Could you check a few things on this drawing? It's one solid part, dimensions in mm from its lowest x, y, z. A direction names the side the tool comes from. Give positions to 0.01 mm unless a question says otherwise; leave off trailing zeros. Loops run counter-clockwise (first coordinate to the right, second up) from the corner with the lowest first, then second, coordinate; pieces in that order, holes last. Notation, with made-up numbers: (-35, 15.25) -> (20, 15.25) arc R15 ccw to (20, 32.25) -> close; hole circle Ø4 at (15.5, 60). An arc over 180 degrees is marked (long way). Use CSV: the item, a comma, the result in double quotes.
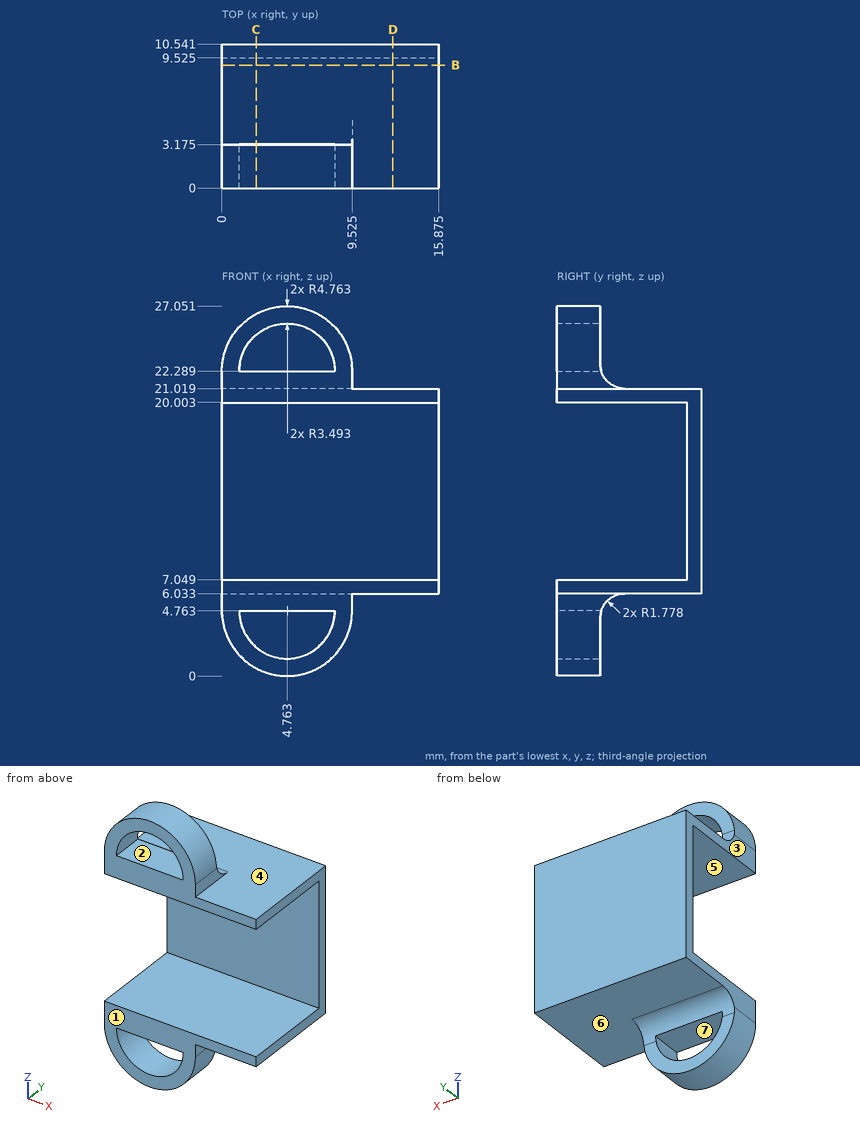
(1) If we section it at B-B, the plane y = 9: Write out the boundary of the cut face in (x, z) (1 decimal).
Answer sheet:
outline,"(0, 6) -> (15.9, 6) -> (15.9, 7) -> (0, 7) -> close; (0, 20) -> (15.9, 20) -> (15.9, 21) -> (0, 21) -> close"
(2) We'd pull the mould along X, two halves only. Please class the marked faces 1, 2 and 3: released by +X, released by -X, zero draft, split by the parting line, or undercut.
Answer sheet:
face 1,"zero draft"
face 2,"undercut"
face 3,"released by -X"
(3) If I drill on L1, parallel to Z at x = 2.25, y = 8; L2, parallel to Y at x = 9.25, z = 13.5 (1 decimal); L3, parallel to Y at x = 8, z = 24.25 (1 decimal), over which ranges is the centre line in solid material (lowest first)? Write a range as from..to.
Answer sheet:
L1,"z = 6.03..7.05, 20..21.02"
L2,"y = 9.5..10.5"
L3,"y = 0..3.2"
(4) Will these pins go through, and if not, where does the flat tip stop? pin 1 Ø5 at (x, y) = (11.5, 6.5) entering from -Z; pin 2 Ø1.5 at (x, z) = (11, 18.5) entering from -Y (1 decimal); pin 3 Ø2 at (x, y) = (6.5, 5) entering from +Z (1 decimal).
Answer sheet:
pin 1,"stops at z = 6.03"
pin 2,"stops at y = 9.5"
pin 3,"stops at z = 21.3"
(5) Which directions (+Z, -Z, +X, -X, +Y, -Y) give clear straight access to the entire face, cutting with the end or side of a thin tool? Please do the marked faces 4, 5, 6 and 7.
Answer sheet:
face 4,"+Z, +X, +Y"
face 5,"+X, -X, -Y"
face 6,"-Z, +X, +Y"
face 7,"+Y, -Y"
(6) If we section it at C-C, the plane x = 2.5: Give the number of separate pieces and of enclosed holes in the cut face.
Answer sheet:
separate pieces,"3"
enclosed holes,"0"
(7) If we section it at D-D, the plane x = 12.5: Write out the boundary of the cut face in (y, z) (1 decimal).
Answer sheet:
outline,"(0, 6) -> (10.5, 6) -> (10.5, 21) -> (0, 21) -> (0, 20) -> (9.5, 20) -> (9.5, 7) -> (0, 7) -> close"
